```python
from build123d import *

# Parameters (mm, degrees)
SKETCH1_W           = 183.134
SKETCH1_H           = 95.25
SKETCH1_W_2         = 13.97
SKETCH1_H_2         = 13.97
BOSS_EXTRUDE1_DEPTH = 1.524


with BuildPart() as part:
    # Sketch1 → Boss-Extrude1 (new body)
    with BuildSketch(Plane(origin=(0, 0, 0), x_dir=(0, 1, 0), z_dir=(0, 0, 1))):
        with Locations((91.567, 47.625)):
            Rectangle(SKETCH1_W, SKETCH1_H)
        with Locations((24.765, 65.913)):
            Rectangle(SKETCH1_W_2, SKETCH1_H_2, mode=Mode.SUBTRACT)
        with Locations((57.785, 65.913)):
            Rectangle(SKETCH1_W_2, SKETCH1_H_2, mode=Mode.SUBTRACT)
        with Locations((90.805, 65.913)):
            Rectangle(SKETCH1_W_2, SKETCH1_H_2, mode=Mode.SUBTRACT)
        with Locations((123.825, 65.913)):
            Rectangle(SKETCH1_W_2, SKETCH1_H_2, mode=Mode.SUBTRACT)
        with Locations((156.845, 65.913)):
            Rectangle(SKETCH1_W_2, SKETCH1_H_2, mode=Mode.SUBTRACT)
        with Locations((57.785, 30.353)):
            Rectangle(SKETCH1_W_2, SKETCH1_H_2, mode=Mode.SUBTRACT)
        with Locations((90.805, 30.353)):
            Rectangle(SKETCH1_W_2, SKETCH1_H_2, mode=Mode.SUBTRACT)
        with Locations((123.825, 30.353)):
            Rectangle(SKETCH1_W_2, SKETCH1_H_2, mode=Mode.SUBTRACT)
        with Locations((156.845, 30.353)):
            Rectangle(SKETCH1_W_2, SKETCH1_H_2, mode=Mode.SUBTRACT)
        with Locations((24.765, 30.353)):
            Rectangle(SKETCH1_W_2, SKETCH1_H_2, mode=Mode.SUBTRACT)
    extrude(amount=BOSS_EXTRUDE1_DEPTH)


solid = part.part
```
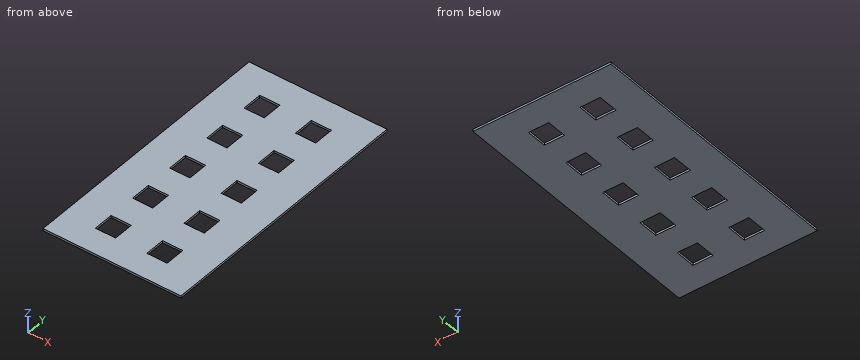
Design review of the part built by this model. Coordinates are the model's own, in mm. Round coordinates to 2 decimals unless told otherwise and drop trailing zeros. Write each loop counter-clockwise with the first axis right and the second up, starting at its lowest first coordinate (ties: lowest second). Pieces come first, ordered by that corner, then holes.
Item 1: We need section A-A on y = 125. Write out the cut boundary in (x, z).
Item 2: We need section B-B on z = 0.25. State how many separate pieces and enclosed holes the cut face has, and give its area (3 significant figures).
Item 3: For probe 1 along Y at (x, z) = (-72.5, 0.4); probe 2 along X at (y, z) = (20.5, 0.2), list the stretches that pass through material, from the lowest coordinate up.
Returned:
1. outline: (-95.25, 0) - (-72.9, 0) - (-72.9, 1.52) - (-95.25, 1.52) - close; (-58.93, 0) - (-37.34, 0) - (-37.34, 1.52) - (-58.93, 1.52) - close; (-23.37, 0) - (0, 0) - (0, 1.52) - (-23.37, 1.52) - close
2. separate pieces: 1
2. enclosed holes: 10
2. area: 15,500 mm2
3. probe 1: y = 0 to 17.78, 31.75 to 50.8, 64.77 to 83.82, 97.79 to 116.84, 130.81 to 149.86, 163.83 to 183.13
3. probe 2: x = -95.25 to -72.9, -58.93 to -37.34, -23.37 to 0
